Source: three-view drawing plus pictorial views. Frame: mm from the lowest corner of the part. Round coordinates to 2 decimals unless told otherwise and drop trailing zeros. Write each loop counter-clockwise with the first axis right and the second up, starting at its lowest first coordinate (ties: lowest second). Pieces come first, ordered by that corner, then holes.
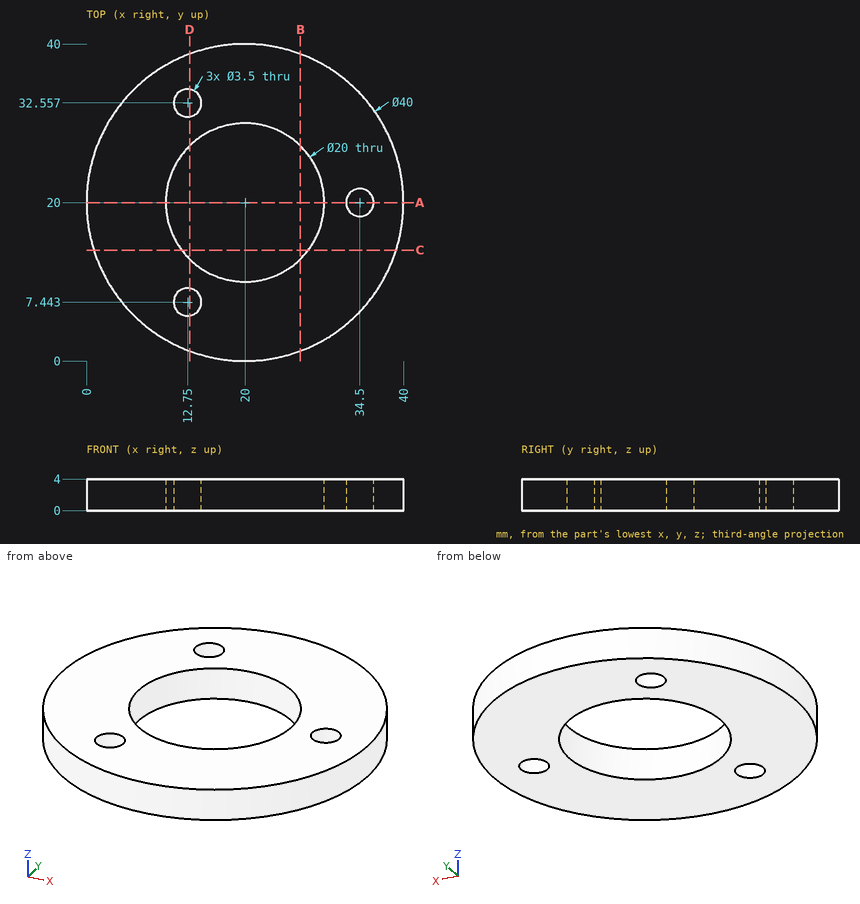
1) Section A-A on y = 20. Output: boundary loops of the cut face in (x, z).
2) Section C-C on y = 14. Output: boundary loops of the cut face in (x, z).
3) Line query: probe 1 along X at (y, z) = (20.5, 3.55); probe 2 along Y at (x, z) = (12.75, 1.4); probe 3 along Y at (x, z) = (20, 1.4). Output: solid intervals per line, ascending.
4) Section D-D on x = 13. Output: boundary loops of the cut face in (y, z) (1 decimal).
5) Section B-B on x = 27. Output: boundary loops of the cut face in (y, z) (1 decimal).
6) First-contact query: P1, Ø2, axis at x = 5, z = 3.5, coming from the +Y side; P2, Ø5, axis at x = 5, y = 23, coming from the -Z side; P3, Ø12, axis at x = 20, y = 20, coming from the -Z side. Flat tips, straight axial feed; report the tip coordinate or a pass-through.
Filled in:
1. outline: (0, 0) - (10, 0) - (10, 4) - (0, 4) - close; (30, 0) - (32.75, 0) - (32.75, 4) - (30, 4) - close; (36.25, 0) - (40, 0) - (40, 4) - (36.25, 4) - close
2. outline: (0.92, 0) - (12, 0) - (12, 4) - (0.92, 4) - close; (28, 0) - (39.08, 0) - (39.08, 4) - (28, 4) - close
3. probe 1: x = 0.01 to 10.01, 29.99 to 32.82, 36.18 to 39.99
3. probe 2: y = 1.36 to 5.69, 9.19 to 13.11, 26.89 to 30.81, 34.31 to 38.64
3. probe 3: y = 0 to 10, 30 to 40
4. outline: (1.3, 0) - (5.7, 0) - (5.7, 4) - (1.3, 4) - close; (9.2, 0) - (12.9, 0) - (12.9, 4) - (9.2, 4) - close; (27.1, 0) - (30.8, 0) - (30.8, 4) - (27.1, 4) - close; (34.3, 0) - (38.7, 0) - (38.7, 4) - (34.3, 4) - close
5. outline: (1.3, 0) - (12.9, 0) - (12.9, 4) - (1.3, 4) - close; (27.1, 0) - (38.7, 0) - (38.7, 4) - (27.1, 4) - close
6. P1: stops at y = 34.28
6. P2: stops at z = 0
6. P3: passes through
